Geometry check sheet. Reference: drawing and pictorial views, mm from the part's lowest x, y, z. A direction names the side the tool comes from. Coordinates: 2 decimals unless noted, no trailing zeros. Loops run counter-clockwise (first coordinate to the right, second up) from the corner with the lowest first, then second, coordinate; pieces in that order, holes last. Notation, with made-up numbers: (-21, 88.25) -> (-11, 88.25) arc R19 cw to (-11, 100.25) -> close; hole circle Ø5 at (51, -28). An arc over 180 degrees is marked (long way). Use one line per item in the form item = value.
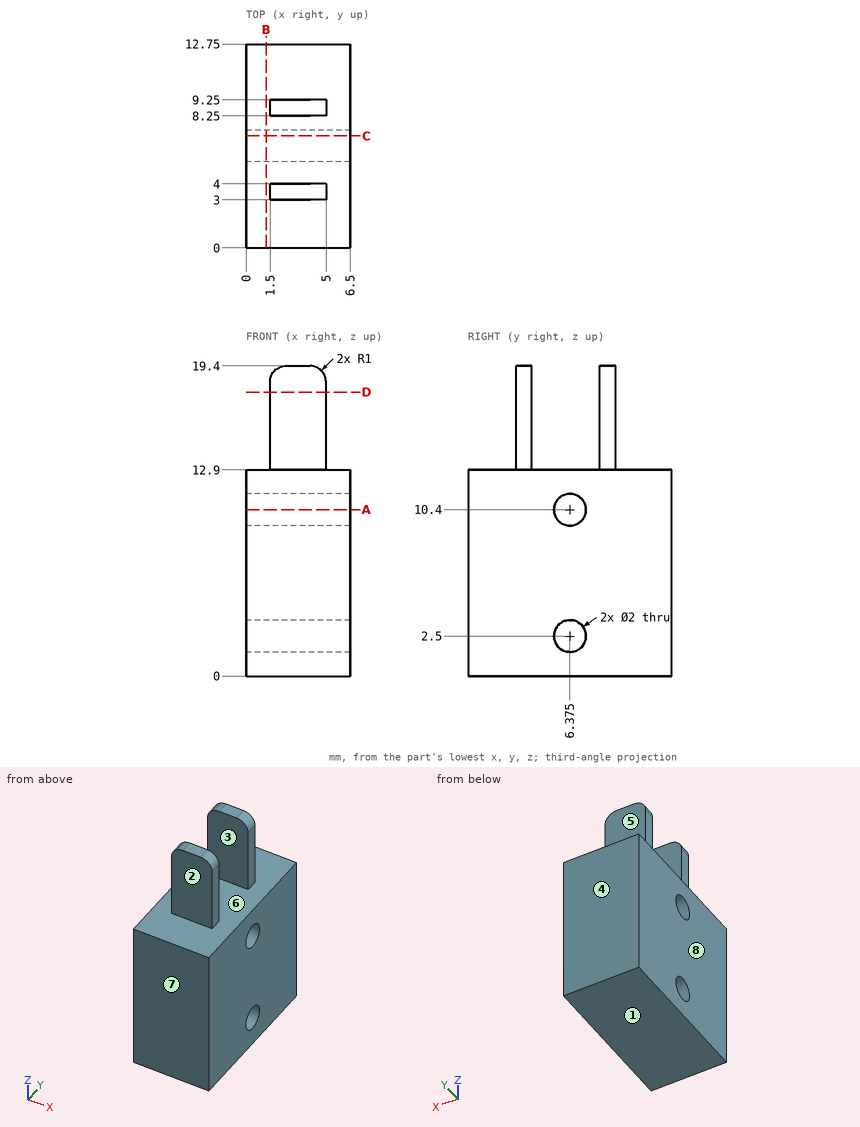
(1) Section check B-B, the plane x = 1.25. Record the boundary of the cut face in (y, z) (3 decimals), plus the area to 3 significant figures.
Established:
outline = (0, 0) -> (12.75, 0) -> (12.75, 12.9) -> (0, 12.9) -> close; hole circle Ø2 at (6.375, 2.5); hole circle Ø2 at (6.375, 10.4)
area = 158 mm²
(2) Section check A-A, the plane z = 10.4. Record the boundary of the cut face in (x, y) (3 decimals).
Established:
outline = (0, 0) -> (6.5, 0) -> (6.5, 5.375) -> (0, 5.375) -> close; (0, 7.375) -> (6.5, 7.375) -> (6.5, 12.75) -> (0, 12.75) -> close
(3) Mould release check, pull along Y, two halves, no side actions. Record for the marked faces 6, 7 and 8: +Y half, -Y half, draft (parallel to the pull), parting line (faces both ways), or undercut.
Established:
face_6 = undercut
face_7 = -Y half
face_8 = draft
(4) Scan lines: line 1 along Y through (x, z) = (4.5, 18); line 2 along Y through (x, z) = (2.25, 10.4) (3 decimals); line 3 along Z through (x, y) = (2, 6.25). Record each from-to range of solid material in increasing order.
Established:
line_1 = 3 to 4, 8.25 to 9.25
line_2 = 0 to 5.375, 7.375 to 12.75
line_3 = 0 to 1.51, 3.49 to 9.41, 11.39 to 12.9
(5) Go/stop test with flat-tipped pins: P1, Ø0.5, axis at y = 8.5, z = 17, coming from the +X side; P2, Ø1.8, axis at x = 3.5, z = 16.5, coming from the +Y side; P3, Ø1, axis at x = 2.5, z = 17.5, coming from the -Y side. Record where each tip stops, or that it passes through.
Established:
P1 = 5
P2 = 9.25
P3 = 3
(6) Tool access check on the marked faces 1, 2, 3, 4 and 5. Record the directions out of +Z, -Z, +X, -X, +Y, -Y that give a thin tool (end or side, any length) a straight path to the whole face; none if there is none.
Established:
face_1 = -Z, +X, -X, +Y, -Y
face_2 = +Z, +X, -X, -Y
face_3 = +Z, +X, -X
face_4 = +Z, -Z, +X, -X, +Y
face_5 = +Z, +X, -X, +Y
(7) Section check C-C, the plane y = 7. Record the boundary of the cut face in (x, z).
Established:
outline = (0, 0) -> (6.5, 0) -> (6.5, 1.72) -> (0, 1.72) -> close; (0, 3.28) -> (6.5, 3.28) -> (6.5, 9.62) -> (0, 9.62) -> close; (0, 11.18) -> (6.5, 11.18) -> (6.5, 12.9) -> (0, 12.9) -> close
(8) Section check D-D, the plane z = 17.75. Record the boundary of the cut face in (x, y).
Established:
outline = (1.5, 3) -> (5, 3) -> (5, 4) -> (1.5, 4) -> close; (1.5, 8.25) -> (5, 8.25) -> (5, 9.25) -> (1.5, 9.25) -> close
